Design review of the part built by this model. Coordinates are the model's own, in mm. Face numbers are marked on the shaded views. A direction names the side the tool comes from. Coordinates: 2 decimals unless noted, no trailing zeros. Loops run counter-clockwise (first coordinate to the right, second up) from the corner with the lowest first, then second, coordinate; pieces in that order, holes last. Notation, with made-up numbers: (58.25, 11.5) - (77.25, 11.5) arc R16 cw to (77.25, 28.5) - close; hole circle Ø3 at (70.5, 11.25). An arc over 180 degrees is marked (long way). Answer in a Markdown table with one row per item. Add a question column.
(1) For the marked faces 1, 2, 3, 4 and 5, list the 3-axis set-ups (+Z, -Z, +X, -X, +Y, -Y) from which the entire face can be reached by the end or side of a thin tool; tool diameter is ignored.
(2) Clearance check with flat-ended pins moving along their axes: pin 1 (6.5 mm diameter, centred on y = 2.5, z = 17.5, fed in from +X); pin 2 (4.5 mm diameter, centred on x = 16.53, y = 20.96, fed in from +Z); pin 3 (4 mm diameter, centred on x = 38, z = 17, fed in from +Y) (3 decimals); pin 4 (10 mm diameter, centred on y = 1, z = 17, fed in from -X). State where each tip first meets the part, or that it passes through.
(3) We need section B-B, the plane z = 2.75. Write out the cut boundary in (x, y) (3 decimals), plus the area to 3 significant figures.
(4) The part is to be moulded in two halves that separate along X. For the marked faces 6, 7 and 8, say which applies: released by +X, released by -X, zero draft, split by the parting line, or undercut.
(5) We need section C-C, the plane x = 27.5. Write out the cut boundary in (y, z).
(6) We need section A-A, the plane y = 0. Write out the cut boundary in (x, z), plus the area to 3 significant figures.
(7) To check wall thickness, follow L1, parallel to Y at x = 56.5, z = 19.5; L2, parallel to Y at x = 57, z = 3.25; L3, parallel to X at y = -23, z = 9.5. State the ranges of each line that lie inside material, in increasing order. Write a range as [from, to].
from build123d import *

# Parameters (mm, degrees)
F0_R     = 2.921
F0_R_2   = 12.7
F1_DEPTH = 25.4


# Not quite as in the source:
# - the program builds the solid bodies; features that only make, move or delete a surface that nothing else refers to are left out


with BuildPart() as f1:
    # F0 (on Top) → F1 (new body)
    with BuildSketch(Plane.XY):
        Polygon((31.1358614907, 25.4), (12.0858614907, 25.4), (12.0858614907, 6.35), (16.5308614907, 6.35), (16.5308614907, -6.35), (12.0858614907, -6.35), (12.0858614907, -25.4), (31.1358614907, -25.4), (31.1358614907, -20.955), (43.8358614907, -20.955), (43.8358614907, -25.4), (62.8858614907, -25.4), (62.8858614907, -6.35), (58.4408614907, -6.35), (58.4408614907, 6.35), (62.8858614907, 6.35), (62.8858614907, 25.4), (43.8358614907, 25.4), (43.8358614907, 20.955), (31.1358614907, 20.955), align=None)
        with Locations((16.5308614907, -20.955)):
            Circle(F0_R, mode=Mode.SUBTRACT)
        with Locations((37.4858614907, 0)):
            Circle(F0_R_2, mode=Mode.SUBTRACT)
        with Locations((58.4408614907, -20.955)):
            Circle(F0_R, mode=Mode.SUBTRACT)
        with Locations((16.5308614907, 20.955)):
            Circle(F0_R, mode=Mode.SUBTRACT)
        with Locations((58.4408614907, 20.955)):
            Circle(F0_R, mode=Mode.SUBTRACT)
    extrude(amount=F1_DEPTH)


solid = f1.part
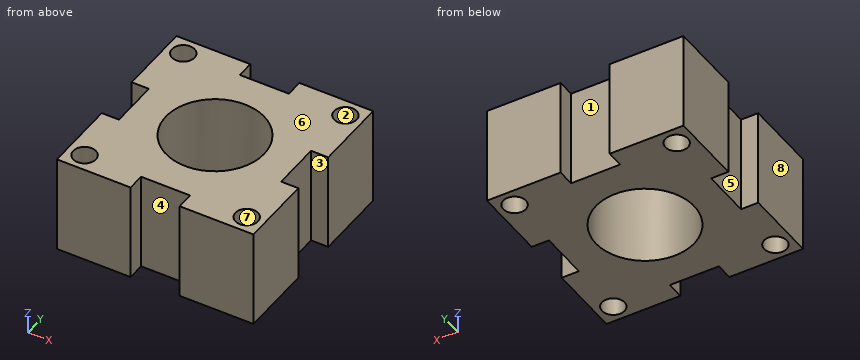
Responses:
| question | item | result |
|---|---|---|
| 1 | face 1 | +Z, -Z, +Y |
| 1 | face 2 | +Z, -Z |
| 1 | face 3 | +Z, -Z, +X |
| 1 | face 4 | +Z, -Z, -Y |
| 1 | face 5 | +Z, -Z, -X |
| 2 | pin 1 | stops at x = 58.44 |
| 2 | pin 2 | passes through |
| 2 | pin 3 | stops at y = 20.955 |
| 2 | pin 4 | stops at x = 16.53 |
| 3 | outline | (12.086, -25.4) - (31.136, -25.4) - (31.136, -20.955) - (43.836, -20.955) - (43.836, -25.4) - (62.886, -25.4) - (62.886, -6.35) - (58.441, -6.35) - (58.441, 6.35) - (62.886, 6.35) - (62.886, 25.4) - (43.836, 25.4) - (43.836, 20.955) - (31.136, 20.955) - (31.136, 25.4) - (12.086, 25.4) - (12.086, 6.35) - (16.531, 6.35) - (16.531, -6.35) - (12.086, -6.35) - close; hole circle Ø5.842 at (16.531, -20.955); hole circle Ø5.842 at (16.531, 20.955); hole circle Ø25.4 at (37.486, 0); hole circle Ø5.842 at (58.441, -20.955); hole circle Ø5.842 at (58.441, 20.955) |
| 3 | area | 1,740 mm2 |
| 4 | face 6 | zero draft |
| 4 | face 7 | undercut |
| 4 | face 8 | released by -X |
| 5 | outline | (-25.4, 0) - (-7.85, 0) - (-7.85, 25.4) - (-25.4, 25.4) - close; (7.85, 0) - (25.4, 0) - (25.4, 25.4) - (7.85, 25.4) - close |
| 6 | outline | (16.53, 0) - (24.79, 0) - (24.79, 25.4) - (16.53, 25.4) - close; (50.19, 0) - (58.44, 0) - (58.44, 25.4) - (50.19, 25.4) - close |
| 6 | area | 419 mm2 |
| 7 | L1 | y = [-25.4, -23.14], [-18.77, 18.77], [23.14, 25.4] |
| 7 | L2 | y = [-25.4, -23.5], [-18.41, 18.41], [23.5, 25.4] |
| 7 | L3 | x = [12.09, 14.45], [18.62, 31.14], [43.84, 56.36], [60.53, 62.89] |
